Check sheet for the drawn part. Datum: minimum x, y, z corner. Units: mm. A direction names the side the tool comes from. Give positions to 0.01 mm unless a question says otherwise; leave off trailing zeros. Order: outer loops, then holes, each group sorted by start corner. A loop starts at its lowest first (then second) coordinate and runs counter-clockwise, first axis right, second up.
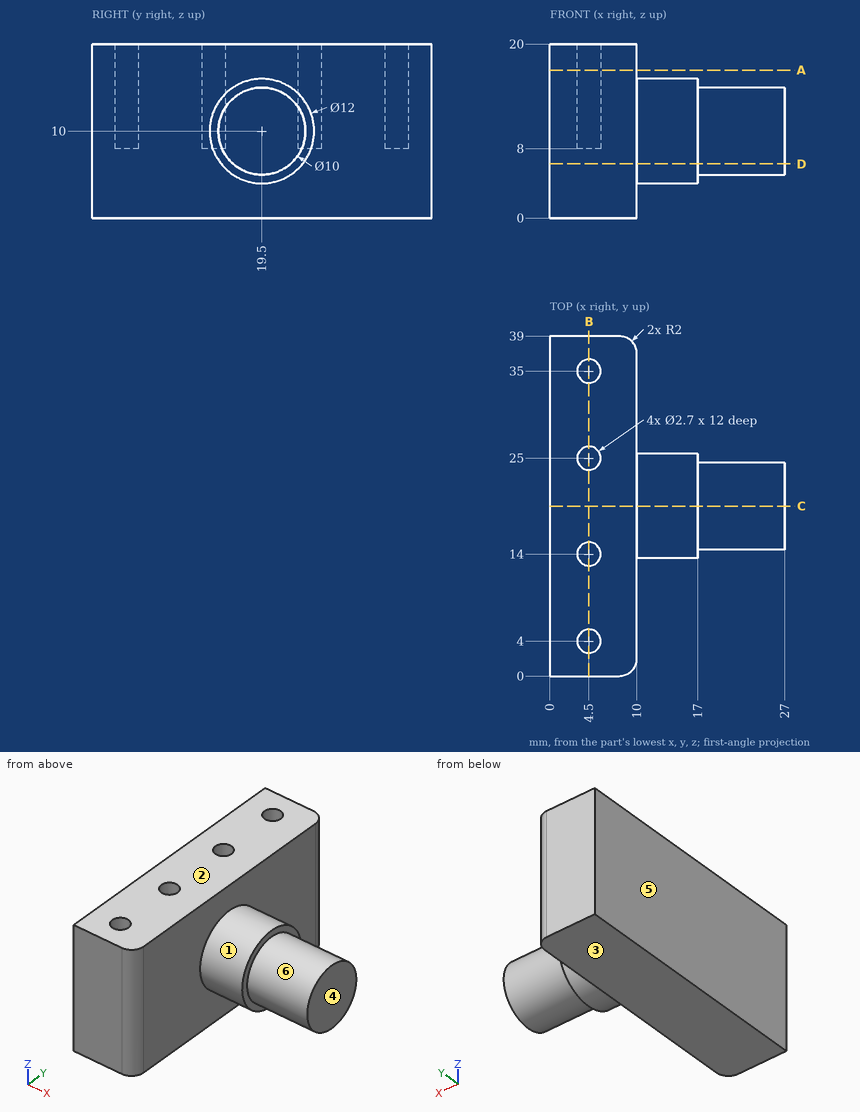
(1) Section check B-B, the plane x = 4.5. Enter the section's corners in (y, z), then the cut area to 3 significant figures.
Solved:
outline: (0, 0) - (39, 0) - (39, 20) - (36.35, 20) - (36.35, 8) - (33.65, 8) - (33.65, 20) - (26.35, 20) - (26.35, 8) - (23.65, 8) - (23.65, 20) - (15.35, 20) - (15.35, 8) - (12.65, 8) - (12.65, 20) - (5.35, 20) - (5.35, 8) - (2.65, 8) - (2.65, 20) - (0, 20) - close
area: 650 mm2
(2) Section check D-D, the plane z = 6.25. Enter the section's corners in (x, y), then the cut area to 3 significant figures.
Solved:
outline: (0, 0) - (8, 0) arc R2 ccw to (10, 2) - (10, 14.82) - (17, 14.82) - (17, 16.19) - (27, 16.19) - (27, 22.81) - (17, 22.81) - (17, 24.18) - (10, 24.18) - (10, 37) arc R2 ccw to (8, 39) - (0, 39) - close
area: 520 mm2
(3) Set-up check for the marked faces 5 and 6: record each of +Z, -Z, +X, -X, +Y, -Y from which the full face is reachable in a straight line by a thin tool's end or side.
Solved:
face 5: +Z, -Z, -X, +Y, -Y
face 6: +X
(4) Scan lines: line 1 (Y direction, x = 4.5, z = 17); line 2 (X direction, y = 32, z = 9.5); line 3 (X direction, y = 34.5, z = 12.5). Record each from-to range of solid material in increasing order.
Solved:
line 1: y = 0 to 2.65, 5.35 to 12.65, 15.35 to 23.65, 26.35 to 33.65, 36.35 to 39
line 2: x = 0 to 10
line 3: x = 0 to 3.25, 5.75 to 10
(5) Section check C-C, the plane y = 19.5. Enter the section's corners in (x, z), then the cut area to 3 significant figures.
Solved:
outline: (0, 0) - (10, 0) - (10, 4) - (17, 4) - (17, 5) - (27, 5) - (27, 15) - (17, 15) - (17, 16) - (10, 16) - (10, 20) - (0, 20) - close
area: 384 mm2
(6) Go/stop test with flat-tipped pins: pin 1 (0.8 mm diameter, centred on x = 4, y = 35.5, fed in from +Z); pin 2 (2 mm diameter, centred on x = 4.5, y = 25.5, fed in from +Z); pin 3 (1 mm diameter, centred on x = 21, y = 24.5, fed in from -Z); pin 4 (1 mm diameter, centred on x = 11, y = 16, fed in from +Z). Record where each tip stops, or that it passes through.
Solved:
pin 1: stops at z = 8
pin 2: stops at z = 20
pin 3: stops at z = 7.82
pin 4: stops at z = 15.2
(7) Release check for a two-part mould opening along Z. For the marked faces 1, 2, 3 and 4 record: pulls with the +Z half, pulls with the -Z half, needs draft (parallel to the pull), parting line crosses it, or undercut.
Solved:
face 1: parting line crosses it
face 2: pulls with the +Z half
face 3: pulls with the -Z half
face 4: needs draft
(8) Section check A-A, the plane z = 17. Enter the section's corners in (x, y).
Solved:
outline: (0, 0) - (8, 0) arc R2 ccw to (10, 2) - (10, 37) arc R2 ccw to (8, 39) - (0, 39) - close; hole circle Ø2.7 at (4.5, 4); hole circle Ø2.7 at (4.5, 14); hole circle Ø2.7 at (4.5, 25); hole circle Ø2.7 at (4.5, 35)
